Design review of the part shown in the three views and the two pictorial views. Dimensions are in mm from the part's minimum x, y and z. Round coordinates to 2 decimals unless told otherwise and drop trailing zeros. Write each loop counter-clockwise with the first axis right and the second up, starting at its lowest first coordinate (ties: lowest second). Pieces come first, ordered by that corner, then holes. Notation, with made-up numbers: (39.5, 22.5) -> (49.5, 22.5) arc R33 ccw to (49.5, 60.5) -> close; hole circle Ø8 at (-6.75, -34.5). An arc over 180 degrees is marked (long way). Answer as a JSON object with one key per item and string values. Group by question number.
1) We need section C-C, the plane z = 0.25. Write out the cut boundary in (x, y).
2) We need section B-B, the plane y = 110. Write out the cut boundary in (x, z).
3) We need section D-D, the plane x = 3.5. Write out the cut boundary in (y, z), then the cut area to 3 significant figures.
4) We need section A-A, the plane x = 10. Write out the cut boundary in (y, z).
5) To check wall thickness, follow probe 1 along Y at (x, z) = (10, 0.7); probe 2 along Y at (x, z) = (9, 0.5); probe 3 along Y at (x, z) = (15.75, 0.15). State the ranges of each line that lie inside material, in increasing order. Write a range as [from, to].
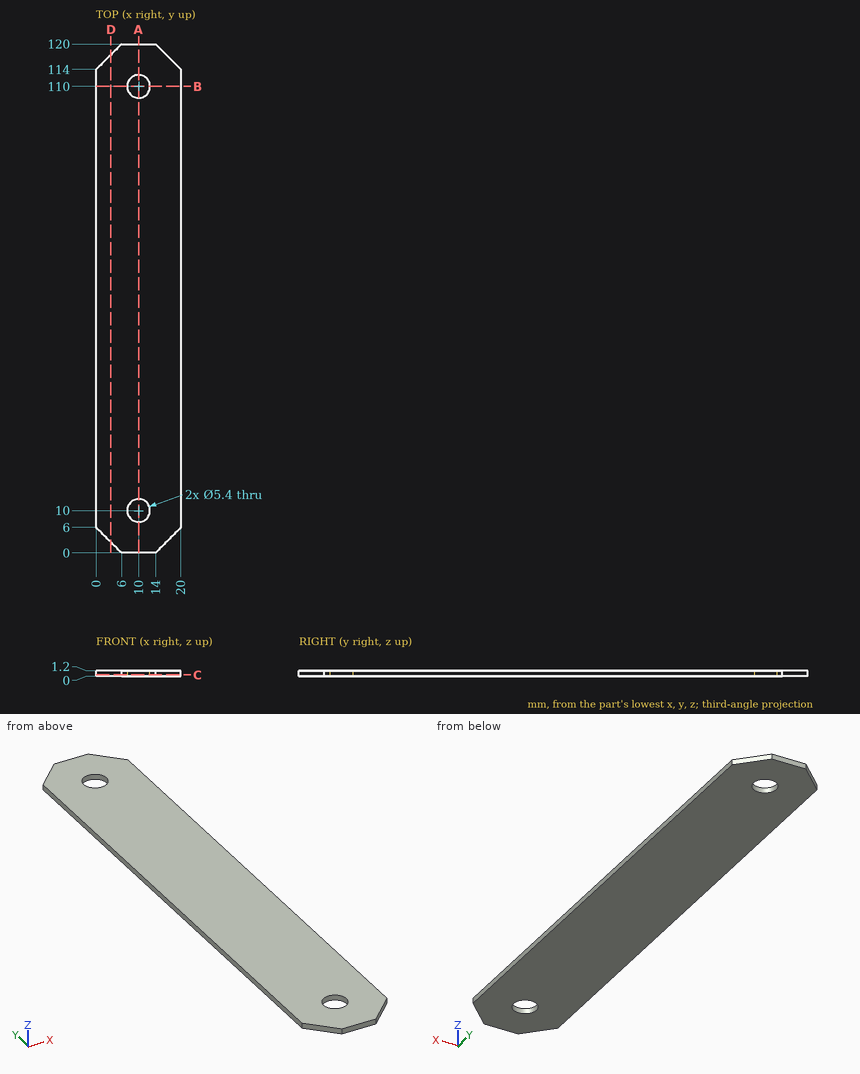
Here are the results:
{
 "1": {"outline": "(0, 6) -> (6, 0) -> (14, 0) -> (20, 6) -> (20, 114) -> (14, 120) -> (6, 120) -> (0, 114) -> close; hole circle Ø5.4 at (10, 10); hole circle Ø5.4 at (10, 110)"},
 "2": {"outline": "(0, 0) -> (7.3, 0) -> (7.3, 1.2) -> (0, 1.2) -> close; (12.7, 0) -> (20, 0) -> (20, 1.2) -> (12.7, 1.2) -> close"},
 "3": {"outline": "(2.5, 0) -> (117.5, 0) -> (117.5, 1.2) -> (2.5, 1.2) -> close", "area": "138 mm^2"},
 "4": {"outline": "(0, 0) -> (7.3, 0) -> (7.3, 1.2) -> (0, 1.2) -> close; (12.7, 0) -> (107.3, 0) -> (107.3, 1.2) -> (12.7, 1.2) -> close; (112.7, 0) -> (120, 0) -> (120, 1.2) -> (112.7, 1.2) -> close"},
 "5": {"probe 1": "y = [0, 7.3], [12.7, 107.3], [112.7, 120]", "probe 2": "y = [0, 7.49], [12.51, 107.49], [112.51, 120]", "probe 3": "y = [1.75, 118.25]"}
}
